```python
from build123d import *

# Parameters (mm, degrees)
SKETCH1_W           = 11.5
SKETCH1_H           = 8
BOSS_EXTRUDE1_DEPTH = 13.3
CUT_EXTRUDE1_REACH  = 20.032
SKETCH2_R           = 2.125
CUT_EXTRUDE2_REACH  = 20.032
CUT_EXTRUDE3_REACH  = 18.552
SKETCH4_W           = 8
SKETCH4_H           = 11.55
CUT_EXTRUDE4_REACH  = 17.032
SKETCH5_R           = 2.125
FILLET1_R           = 0.5


with BuildPart() as part:
    # Sketch1 → Boss-Extrude1 (new body)
    with BuildSketch(Plane(origin=(0, 0, 0), x_dir=(1, 0, 0), z_dir=(0, 1, 0))):
        Rectangle(SKETCH1_W, SKETCH1_H)
    extrude(amount=BOSS_EXTRUDE1_DEPTH)

    # Sketch2 → Cut-Extrude1 (cut, up to next)
    with BuildSketch(Plane(origin=(5.75, 0, 0), x_dir=(0, 0, -1), z_dir=(1, 0, 0)), mode=Mode.PRIVATE) as cut_extrude1_sk1:
        with Locations((0, 9.3)):
            Circle(SKETCH2_R)
    cut_extrude1_tool1 = extrude(cut_extrude1_sk1.sketch, amount=-CUT_EXTRUDE1_REACH, mode=Mode.PRIVATE) & part.part
    add(cut_extrude1_tool1.solids().sort_by_distance((5.75, 9.3, 0))[0], mode=Mode.SUBTRACT)

    # Sketch3 → Cut-Extrude2 (cut, up to next)
    with BuildSketch(Plane(origin=(5.75, 0, 0), x_dir=(0, 0, -1), z_dir=(1, 0, 0)), mode=Mode.PRIVATE) as cut_extrude2_sk1:
        with BuildLine():
            Line((4, 13.3), (0, 13.3))
            ThreePointArc((0, 13.3), (2.828427125, 12.128427125), (4, 9.3))
            Line((4, 9.3), (4, 13.3))
        make_face()
    cut_extrude2_tool1 = extrude(cut_extrude2_sk1.sketch, amount=-CUT_EXTRUDE2_REACH, mode=Mode.PRIVATE) & part.part
    # Sketch3 → Cut-Extrude2 (cut, up to next)
    with BuildSketch(Plane(origin=(5.75, 0, 0), x_dir=(0, 0, -1), z_dir=(1, 0, 0)), mode=Mode.PRIVATE) as cut_extrude2_sk2:
        with BuildLine():
            Line((0, 13.3), (-4, 13.3))
            Line((-4, 13.3), (-4, 9.3))
            ThreePointArc((-4, 9.3), (-2.828427125, 12.128427125), (0, 13.3))
        make_face()
    cut_extrude2_tool2 = extrude(cut_extrude2_sk2.sketch, amount=-CUT_EXTRUDE2_REACH, mode=Mode.PRIVATE) & part.part
    add(cut_extrude2_tool1.solids().sort_by_distance((5.75, 12.406528, -3.106528))[0], mode=Mode.SUBTRACT)
    add(cut_extrude2_tool2.solids().sort_by_distance((5.75, 12.406528, 3.106528))[0], mode=Mode.SUBTRACT)

    # Sketch4 → Cut-Extrude3 (cut, up to next)
    with BuildSketch(Plane.XY.offset(4), mode=Mode.PRIVATE) as cut_extrude3_sk1:
        with Locations((0, 7.525)):
            Rectangle(SKETCH4_W, SKETCH4_H)
    cut_extrude3_tool1 = extrude(cut_extrude3_sk1.sketch, amount=-CUT_EXTRUDE3_REACH, mode=Mode.PRIVATE) & part.part
    add(cut_extrude3_tool1.solids().sort_by_distance((0, 7.525, 4))[0], mode=Mode.SUBTRACT)

    # Sketch5 → Cut-Extrude4 (cut, up to next)
    with BuildSketch(Plane.XZ, mode=Mode.PRIVATE) as cut_extrude4_sk1:
        with Locations(Location((0, 0, 0), (0, 0, 270))):
            Circle(SKETCH5_R)
    cut_extrude4_tool1 = extrude(cut_extrude4_sk1.sketch, amount=-CUT_EXTRUDE4_REACH, mode=Mode.PRIVATE) & part.part
    add(cut_extrude4_tool1.solids().sort_by_distance((0, 0, 0))[0], mode=Mode.SUBTRACT)

    # Fillet1
    fillet1_edges = [part.edges().sort_by_distance(p)[0] for p in [
        (5.75, 0, 0),
        (-5.75, 0, 0),
    ]]
    fillet(fillet1_edges, radius=FILLET1_R)


solid = part.part
```
Geometry: final body of the model. Coordinates: model frame, mm. A direction names the side the tool comes from. Coordinates: 2 decimals unless noted, no trailing zeros. Write each loop counter-clockwise with the first axis right and the second up, starting at its lowest first coordinate (ties: lowest second). Pieces come first, ordered by that corner, then holes. Notation, with made-up numbers: M -32,-40 L -7,-40 A9 ccw -7,-30 Z; hole C 54.5,31.5 d8. An arc over 180 degrees is marked long. Answer as CSV lines item,"result". Start each with the question number.
Q1. Cut plane A-A on x = 0. Return the cut outline in (y, z) (3 decimals), then the cut area to 3 significant figures.
Q2. Mould query, pull axis Y, two halves, no side actions, for faces 1 (the flat face through (4, 6, 0)), 2 (the flat face through (2.3, 0, -0.1)), 3 (the cylindrical face through (4.887, 11.407, 0.277)), 4 (the cylindrical face through (-4.863, 11.407, 0.277)). Classes: released by +Y, released by -Y, zero draft, split by the parting line, or undercut.
Q3. Cut plane C-C on z = -0.75. Return the cut outline in (x, y), then the cut area to 3 significant figures.
Q4. Reachability of faces 5 (the flat face through (5.75, 5, 0)), 6 (the flat face through (-2, 1.75, -2)) from +Z, -Z, +X, -X, +Y, -Y: full face, straight path, thin tool, end or side. Return the list, or none.
Q5. Cut plane D-D on y = 10.25. Return the cut outline in (x, z), then the cut area to 3 significant figures.
Q6. Cut plane B-B on y = 3.25. Return the cut outline in (x, z).
Q7. Line query: line 1 (Y direction, x = 4.65, z = 0) (3 decimals); line 2 (X direction, y = 5.75, z = -1.25); line 3 (Y direction, x = -0.5, z = 2.25). Output: solid intervals per line, ascending. Write a range as from..to.
Q8. Pin query (flat end, axial travel): P1, Ø4, axis at y = 10, z = -1.5, coming from the +X side; P2, Ø4, axis at y = 9.3, z = 0, coming from the -X side; P3, Ø2, axis at x = -1, z = 1, coming from the +Y side. Return the tip coordinate at first contact, or that it passes through.
Findings below:
1,outline,"M 0,-4 L 1.75,-4 L 1.75,-2.125 L 0,-2.125 Z; M 0,2.125 L 1.75,2.125 L 1.75,4 L 0,4 Z"
1,area,"6.56 mm2"
2,face 1,"zero draft"
2,face 2,"released by -Y"
2,face 3,"undercut"
2,face 4,"undercut"
3,outline,"M -5.75,0.5 A0.5 ccw -5.25,0 L -1.99,0 L -1.99,1.75 L -4,1.75 L -4,7.31 L -5.75,7.31 Z; M -5.75,11.29 L -4,11.29 L -4,13.23 L -5.75,13.23 Z; M 1.99,0 L 5.25,0 A0.5 ccw 5.75,0.5 L 5.75,7.31 L 4,7.31 L 4,1.75 L 1.99,1.75 Z; M 4,11.29 L 5.75,11.29 L 5.75,13.23 L 4,13.23 Z"
3,area,"39.3 mm2"
4,face 5,"+Z, -Z, +X, +Y, -Y"
4,face 6,"+Z, -Z, +Y"
5,outline,"M -5.75,-3.89 L -4,-3.89 L -4,-1.9 L -5.75,-1.9 Z; M -5.75,1.9 L -4,1.9 L -4,3.89 L -5.75,3.89 Z; M 4,-3.89 L 5.75,-3.89 L 5.75,-1.9 L 4,-1.9 Z; M 4,1.9 L 5.75,1.9 L 5.75,3.89 L 4,3.89 Z"
5,area,"13.9 mm2"
6,outline,"M -5.75,-4 L -4,-4 L -4,4 L -5.75,4 Z; M 4,-4 L 5.75,-4 L 5.75,4 L 4,4 Z"
7,line 1,"y = 0..7.175, 11.425..13.3"
7,line 2,"x = -5.75..-4, 4..5.75"
7,line 3,"y = 0..1.75"
8,P1,"stops at x = 5.75"
8,P2,"passes through"
8,P3,"stops at y = 1.75"
